For this review, take the finished solid that the model builds, in its own axes (mm). Round coordinates to 2 decimals unless told otherwise and drop trailing zeros. Order: outer loops, then holes, each group sorted by start corner. A loop starts at its lowest first (then second) coordinate and runs counter-clockwise, first axis right, second up. Notation, with made-up numbers: (-11.5, 38.5) -> (24.5, 38.5) arc R32 cw to (24.5, 65.5) -> close; hole circle Ø10 at (36.5, 6). An arc over 180 degrees is marked (long way). Answer in a Markdown table with one row per item.
```python
from build123d import *

# Parameters (mm, degrees)
SKETCH1_R           = 3
BOSS_EXTRUDE1_DEPTH = 3


with BuildPart() as part:
    # Sketch1 → Boss-Extrude1 (new body)
    with BuildSketch(Plane.XY):
        Polygon((1018.05312216, -2273.263793346), (1511.008064266, -1681.744203601), (1011.673345649, -1265.613408316), (518.718403543, -1857.132998062), align=None)
        with Locations((701.753786497, -1797.896182314)):
            Circle(SKETCH1_R, mode=Mode.SUBTRACT)
        with Locations((1327.972681313, -1740.981019348)):
            Circle(SKETCH1_R, mode=Mode.SUBTRACT)
        with Locations((1235.174126546, -1714.270941976)):
            Circle(SKETCH1_R, mode=Mode.SUBTRACT)
        with Locations((1278.631701009, -1695.259387021)):
            Circle(SKETCH1_R, mode=Mode.SUBTRACT)
        with Locations((1323.446984512, -1691.186259901)):
            Circle(SKETCH1_R, mode=Mode.SUBTRACT)
        with Locations((697.228089696, -1748.101422866)):
            Circle(SKETCH1_R, mode=Mode.SUBTRACT)
        with Locations((788.216365742, -1754.893596459)):
            Circle(SKETCH1_R, mode=Mode.SUBTRACT)
        with Locations((742.043373199, -1744.028295746)):
            Circle(SKETCH1_R, mode=Mode.SUBTRACT)
        with Locations((751.0947668, -1843.617814641)):
            Circle(SKETCH1_R, mode=Mode.SUBTRACT)
        with Locations((794.552341263, -1824.606259686)):
            Circle(SKETCH1_R, mode=Mode.SUBTRACT)
        with Locations((706.279483297, -1847.690941762)):
            Circle(SKETCH1_R, mode=Mode.SUBTRACT)
        with Locations((1241.510102067, -1783.983605203)):
            Circle(SKETCH1_R, mode=Mode.SUBTRACT)
        with Locations((1332.498378113, -1790.775778796)):
            Circle(SKETCH1_R, mode=Mode.SUBTRACT)
        with Locations((1287.68309461, -1794.848905917)):
            Circle(SKETCH1_R, mode=Mode.SUBTRACT)
        with Locations((940.684020094, -1505.670133727)):
            Circle(SKETCH1_R, mode=Mode.SUBTRACT)
        with Locations((936.610892974, -1460.854850224)):
            Circle(SKETCH1_R, mode=Mode.SUBTRACT)
        with Locations((986.405652422, -1456.329153423)):
            Circle(SKETCH1_R, mode=Mode.SUBTRACT)
        with Locations((1036.200411869, -1451.803456623)):
            Circle(SKETCH1_R, mode=Mode.SUBTRACT)
        with Locations((1040.27353899, -1496.618740126)):
            Circle(SKETCH1_R, mode=Mode.SUBTRACT)
        with Locations((1029.408238276, -1542.791732669)):
            Circle(SKETCH1_R, mode=Mode.SUBTRACT)
        with Locations((959.695575049, -1549.12770819)):
            Circle(SKETCH1_R, mode=Mode.SUBTRACT)
        with Locations((1089.042447715, -2033.207067936)):
            Circle(SKETCH1_R, mode=Mode.SUBTRACT)
        with Locations((1093.115574835, -2078.022351439)):
            Circle(SKETCH1_R, mode=Mode.SUBTRACT)
        with Locations((1043.320815387, -2082.548048239)):
            Circle(SKETCH1_R, mode=Mode.SUBTRACT)
        with Locations((993.52605594, -2087.07374504)):
            Circle(SKETCH1_R, mode=Mode.SUBTRACT)
        with Locations((989.452928819, -2042.258461537)):
            Circle(SKETCH1_R, mode=Mode.SUBTRACT)
        with Locations((1000.318229533, -1996.085468994)):
            Circle(SKETCH1_R, mode=Mode.SUBTRACT)
        with Locations((1070.03089276, -1989.749493473)):
            Circle(SKETCH1_R, mode=Mode.SUBTRACT)
    extrude(amount=BOSS_EXTRUDE1_DEPTH)


solid = part.part
```
Q1. Take a section at B-B, the plane x = 616. Write out the cut boundary in (y, z).
Answer key:
| item | result |
|---|---|
| outline | (-1938.2, 0) -> (-1740.4, 0) -> (-1740.4, 3) -> (-1938.2, 3) -> close |
Q2. Take a section at C-C, the plane y = -2127. Write out the cut boundary in (x, z), then the cut area to 3 significant figures.
Answer key:
| item | result |
|---|---|
| outline | (842.54, 0) -> (1139.95, 0) -> (1139.95, 3) -> (842.54, 3) -> close |
| area | 892 mm^2 |
Q3. Take a section at A-A, the plane z = 0.5. Give the number of separate pieces and of enclosed holes in the cut face, then the cut area to 3 significant figures.
Answer key:
| item | result |
|---|---|
| separate pieces | 1 |
| enclosed holes | 28 |
| area | 500,000 mm^2 |
Q4. Clearance check with flat-ended pins moving along their axes: pin 1 Ø3.5 at (x, y) = (794.55, -1824.61) entering from -Z; pin 2 Ø1.5 at (x, z) = (1062.5, 1.5) entering from -Y; pin 3 Ø1.5 at (y, z) = (-1692, 1.5) entering from -X; pin 4 Ø1.5 at (x, z) = (712, 1.5) entering from -Y. State where each tip first meets the part, or that it passes through.
Answer key:
| item | result |
|---|---|
| pin 1 | passes through |
| pin 2 | stops at y = -2220.83 |
| pin 3 | stops at x = 655.71 |
| pin 4 | stops at y = -2018.83 |
Q5. To check wall thickness, follow probe 1 along Y at (x, z) = (939, 1.75); probe 2 along Y at (x, z) = (957, 0.5); probe 3 along Y at (x, z) = (1322, 1.9). State the ranges of each line that lie inside material, in increasing order.
Answer key:
| item | result |
|---|---|
| probe 1 | y = -2207.38 to -1508.15, -1503.19 to -1462.67, -1459.04 to -1352.82 |
| probe 2 | y = -2222.38 to -1550.44, -1547.81 to -1331.22 |
| probe 3 | y = -1908.54 to -1693.81, -1688.56 to -1524.23 |
